```python
from build123d import *

# Parameters (mm, degrees)
F0_W     = 38.1
F0_H     = 304.8
F1_DEPTH = 3.175
F3_START = 12.7
F2_W     = 304.8
F2_H     = 9.525
F3_DEPTH = 6.35
F4_START = -12.7
F4_DEPTH = 6.35
F6_START = 152.4
F5_W     = 38.1
F5_H     = 12.7
F6_DEPTH = 6.35
F8_START = 9.525
F7_W     = 38.1
F7_H     = 311.15
F8_DEPTH = 3.175


with BuildPart() as f1:
    # F0 (on Top) → F1 (new body)
    with BuildSketch(Plane.XY):
        Rectangle(F0_W, F0_H)
    extrude(amount=F1_DEPTH)

    # F2 (on Right) → F3 (join)
    with BuildSketch(Plane.YZ.offset(F3_START)):
        with Locations((0, 7.9375)):
            Rectangle(F2_W, F2_H)
    extrude(amount=F3_DEPTH)

    # F2 (on Right) → F4 (join)
    with BuildSketch(Plane.YZ.offset(F4_START)):
        with Locations((0, 7.9375)):
            Rectangle(F2_W, F2_H)
    extrude(amount=-F4_DEPTH)

    # F5 (on Front) → F6 (join)
    with BuildSketch(Plane.XZ.offset(F6_START)):
        with Locations((0, 6.35)):
            Rectangle(F5_W, F5_H)
    extrude(amount=F6_DEPTH)

    # F7 (on Top) → F8 (join)
    with BuildSketch(Plane.XY.offset(F8_START)):
        with Locations((0, -3.175)):
            Rectangle(F7_W, F7_H)
        with BuildLine():
            Line((1.5834027278, 127.1139826809), (1.5874468984, -139.7129844058))
            ThreePointArc((1.5874468984, -139.7129844058), (0.0230261009, -141.2873329987), (-1.5864023222, -139.7590247593))
            Line((-1.5864023222, -139.7590247593), (-1.5821546863, 127.1301645063))
            ThreePointArc((-1.5821546863, 127.1301645063), (0.0081149412, 128.587479259), (1.5834027278, 127.1139826809))
        make_face(mode=Mode.SUBTRACT)
    extrude(amount=F8_DEPTH)


solid = f1.part
```
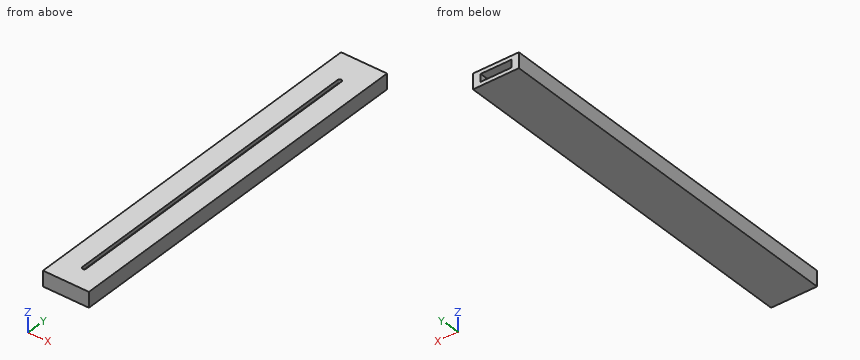
For this review, take the finished solid that the model builds, in its own axes (mm). Give positions to 0.01 mm unless a question says otherwise; leave off trailing zeros. Order: outer loops, then holes, each group sorted by start corner. A loop starts at its lowest first (then second) coordinate and runs counter-clockwise, first axis right, second up.
1) Take a section at A-A (x = 5.5). Give the boundary of the cut face in (y, z) (3 decimals), then the cut area to 3 significant figures.
2) Take a section at C-C (y = 39). Give the boundary of the cut face in (x, z) (3 decimals), then the cut area to 3 significant figures.
3) Insertion check: pin 1 (3 mm diameter, centred on x = 2.5, z = 7.5, fed in from +Y). The pin has a flat end and moves straight along its axis. Give the tip position at first contact, or say it passes through.
4) Wall thickness on line 1 (X direction, y = 26, z = 6); line 2 (Z direction, x = -4, y = -81) (3 decimals); line 3 (Y direction, x = 6, z = 6): over which ranges is each line inside the solid? List them lowest first.
Derived:
1. outline: (-158.75, 0) - (152.4, 0) - (152.4, 3.175) - (-152.4, 3.175) - (-152.4, 9.525) - (152.4, 9.525) - (152.4, 12.7) - (-158.75, 12.7) - close
1. area: 2,020 mm2
2. outline: (-19.05, 0) - (19.05, 0) - (19.05, 12.7) - (1.585, 12.7) - (1.585, 9.525) - (12.7, 9.525) - (12.7, 3.175) - (-12.7, 3.175) - (-12.7, 9.525) - (-1.584, 9.525) - (-1.584, 12.7) - (-19.05, 12.7) - close
2. area: 313 mm2
3. pin 1: stops at y = -152.4
4. line 1: x = -19.05 to -12.7, 12.7 to 19.05
4. line 2: z = 0 to 3.175, 9.525 to 12.7
4. line 3: y = -158.75 to -152.4
